Check sheet for the drawn part. Datum: minimum x, y, z corner. Units: mm. A direction names the side the tool comes from. Coordinates: 2 decimals unless noted, no trailing zeros. Order: outer loops, then holes, each group sorted by start corner. A loop starts at its lowest first (then second) coordinate and runs counter-clockwise, first axis right, second up. Notation, with made-up numbers: (17.25, 79) -> (76.25, 79) arc R25 cw to (76.25, 106) -> close; hole circle Ø3 at (11.5, 32.5). An arc over 180 degrees is marked (long way). Write item = value, one per line. Start each with the question number.
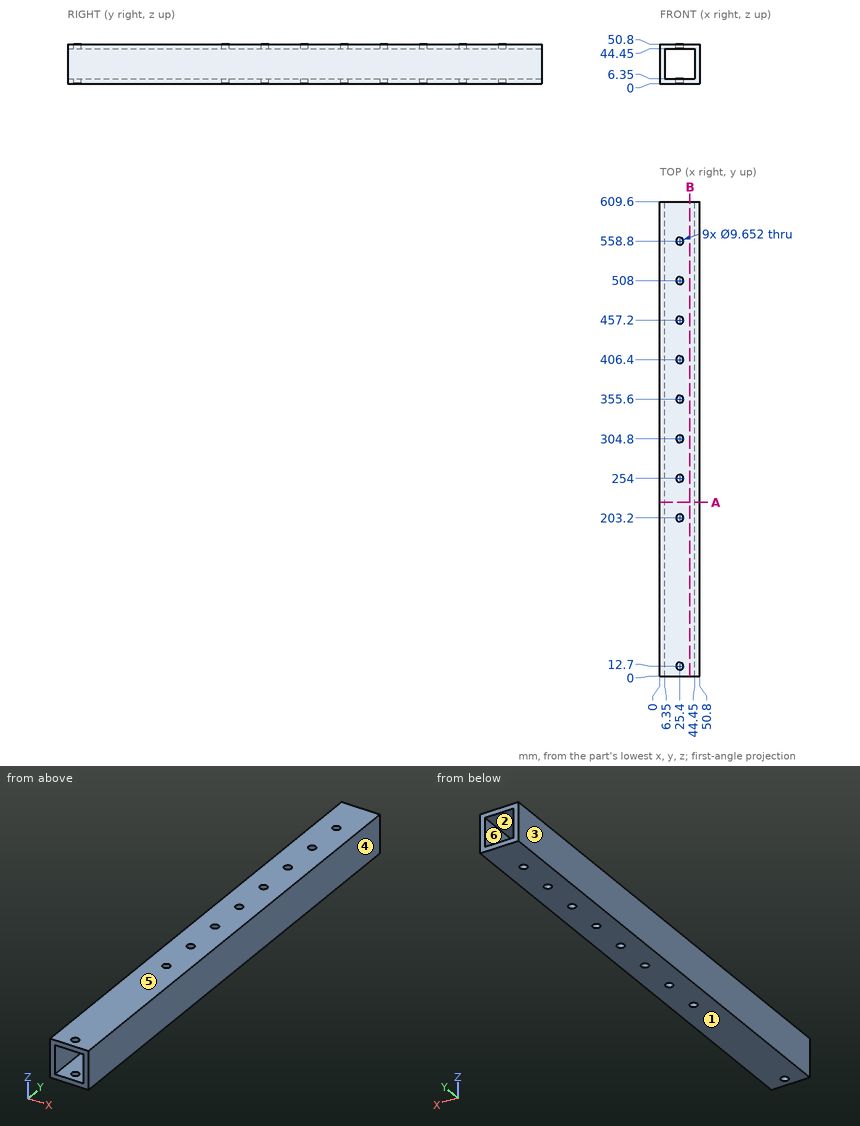
Item 1: Thickness scan on line 1 (X direction, y = 239, z = 14.5); line 2 (X direction, y = 508, z = 2). Record the ranges inside material, lowest first.
Item 2: Mould release check, pull along X, two halves, no side actions. Record for the marked faces 1, 2, 3 and 4: pulls with the +X half, pulls with the -X half, needs draft (parallel to the pull), parting line crosses it, or undercut.
Item 3: Gauge pin test, flat end, axial feed: P1, Ø6, axis at x = 25.4, y = 203.2, coming from the -Z side. Record the tip position at first contact, or that the pin passes through.
Item 4: Section check B-B (x = 38.5). Record the boundary of the cut face in (y, z), then the cut area to 3 significant figures.
Item 5: Section check A-A (y = 223). Record the boundary of the cut face in (x, z).
Item 6: Tool access check on the marked faces 5 and 6. Record the directions out of +Z, -Z, +X, -X, +Y, -Y that give a thin tool (end or side, any length) a straight path to the whole face; none if there is none.
Filled sheet:
q1.line_1 = 0 to 6.35, 44.45 to 50.8
q1.line_2 = 0 to 20.57, 30.23 to 50.8
q2.face_1 = needs draft
q2.face_2 = undercut
q2.face_3 = pulls with the -X half
q2.face_4 = pulls with the +X half
q3.P1 = through
q4.outline = (0, 0) -> (609.6, 0) -> (609.6, 6.35) -> (0, 6.35) -> close; (0, 44.45) -> (609.6, 44.45) -> (609.6, 50.8) -> (0, 50.8) -> close
q4.area = 7,740 mm^2
q5.outline = (0, 0) -> (50.8, 0) -> (50.8, 50.8) -> (0, 50.8) -> close; hole (6.35, 6.35) -> (44.45, 6.35) -> (44.45, 44.45) -> (6.35, 44.45) -> close
q6.face_5 = +Z, +X, -X, +Y, -Y
q6.face_6 = +Y, -Y
